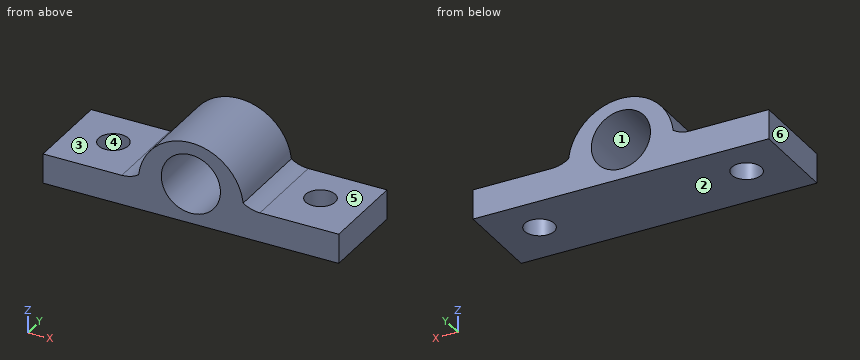
```python
from build123d import *

# Parameters (mm, degrees)
F0_R     = 12.7
F1_DEPTH = 38.1
F2_R     = 6.35
F3_DEPTH = 12.7


with BuildPart() as f1:
    # F0 (on Front) → F1 (new body)
    with BuildSketch(Plane.XZ):
        with BuildLine():
            Line((-63.5, 0), (0, 0))
            Line((0, 0), (63.5, 0))
            Line((63.5, 0), (63.5, 12.7))
            Line((63.5, 12.7), (29.664059, 12.7))
            ThreePointArc((29.664059, 12.7), (25.885674, 13.275075), (22.449471, 14.948219))
            ThreePointArc((22.449471, 14.948219), (0, 35.042593), (-22.449471, 14.948219))
            ThreePointArc((-22.449471, 14.948219), (-25.885674, 13.275075), (-29.664059, 12.7))
            Line((-29.664059, 12.7), (-63.5, 12.7))
            Line((-63.5, 12.7), (-63.5, 0))
        make_face()
        with Locations((0, 17.065845)):
            Circle(F0_R, mode=Mode.SUBTRACT)
    extrude(amount=F1_DEPTH)

    # F2 (on face) → F3 (cut, symmetric)
    with BuildSketch(Plane.XY.offset(12.7)):
        with Locations((-44.45, -17.509114)):
            Circle(F2_R)
        with Locations((44.45, -17.509114)):
            Circle(F2_R)
    extrude(amount=F3_DEPTH, both=True, mode=Mode.SUBTRACT)


solid = f1.part
```
CAD build for the part. Positions are in the model's coordinates, mm. Face numbers are marked on the shaded views. A direction names the side the tool comes from. Round coordinates to 2 decimals unless told otherwise and drop trailing zeros. Loops run counter-clockwise (first coordinate to the right, second up) from the corner with the lowest first, then second, coordinate; pieces in that order, holes last. Notation, with made-up numbers: M 32.5,0 L 76.5,0 A21 cw 76.5,17 Z; hole C 2.25,67.5 d2. An arc over 180 degrees is marked long. Return JSON: item names as keys, results as strings. Group by question number.
(1) Saw through at D-D, the plane z = 27. List the corners of the cut face in (x, y), and give its area (3 significant figures).
(2) Tool access for the marked faces 5 and 6: list every direction of +Z, -Z, +X, -X, +Y, -Y with a clear straight run to the whole face (end or side of a thin tool).
(3) Saw through at B-B, the plane x = 0. List the corners of the cut face in (y, z).
(4) Drop flat-ended pins along their axis: P1, Ø12, axis at y = -19.5, z = 23.5, coming from the +X side; P2, Ø1.5, axis at y = -29.5, z = 26, coming from the +X side; P3, Ø4, axis at x = -38, y = -10.5, coming from the +Z side. Give the stop position or say it passes through.
(5) Wall check: probe 1 along X at (y, z) = (-19, 3); probe 2 along Y at (x, z) = (-44.45, 2.5); probe 3 along X at (y, z) = (-31, 20.5). Give the ranges that are in metal, low to high. Write a range as [from, to].
(6) Saw through at A-A, the plane y = -14. List the corners of the cut face in (x, z), and give its area (3 significant figures).
(7) Mould opens along Z. For the marked faces 1, 2, 3 and 4 say: +Z half, -Z half, draft (parallel to the pull), parting line (faces both ways), or undercut.
(8) Saw through at C-C, the plane z = 6. List the corners of the cut face in (x, y), and give its area (3 significant figures).
Answer list:
{
 "1": {"outline": "M -17.28,-38.1 L -7.91,-38.1 L -7.91,0 L -17.28,0 Z; M 7.91,-38.1 L 17.28,-38.1 L 17.28,0 L 7.91,0 Z", "area": "714 mm2"},
 "2": {"face 5": "+Z, +X, +Y, -Y", "face 6": "+Z, -Z, -X, +Y, -Y"},
 "3": {"outline": "M -38.1,0 L 0,0 L 0,4.37 L -38.1,4.37 Z; M -38.1,29.77 L 0,29.77 L 0,35.04 L -38.1,35.04 Z"},
 "4": {"P1": "x = 22.02", "P2": "x = 18.61", "P3": "z = 12.7"},
 "5": {"probe 1": "[-63.5, -50.62], [-38.28, 38.28], [50.62, 63.5]", "probe 2": "[-38.1, -23.86], [-11.16, 0]", "probe 3": "[-21.11, -12.23], [12.23, 21.11]"},
 "6": {"outline": "M -63.5,0 L -49.74,0 L -49.74,12.7 L -63.5,12.7 Z; M -39.16,0 L 39.16,0 L 39.16,12.7 L 29.66,12.7 A12.7 cw 22.45,14.95 A22.59 ccw -22.45,14.95 A12.7 cw -29.66,12.7 L -39.16,12.7 Z; M 49.74,0 L 63.5,0 L 63.5,12.7 L 49.74,12.7 Z; hole C 0,17.07 d25.4", "area": "1,640 mm2"},
 "7": {"face 1": "undercut", "face 2": "-Z half", "face 3": "+Z half", "face 4": "draft"},
 "8": {"outline": "M -63.5,-38.1 L -6.23,-38.1 L -6.23,0 L -63.5,0 Z; M 6.23,-38.1 L 63.5,-38.1 L 63.5,0 L 6.23,0 Z; hole C -44.45,-17.51 d12.7; hole C 44.45,-17.51 d12.7", "area": "4,110 mm2"}
}
